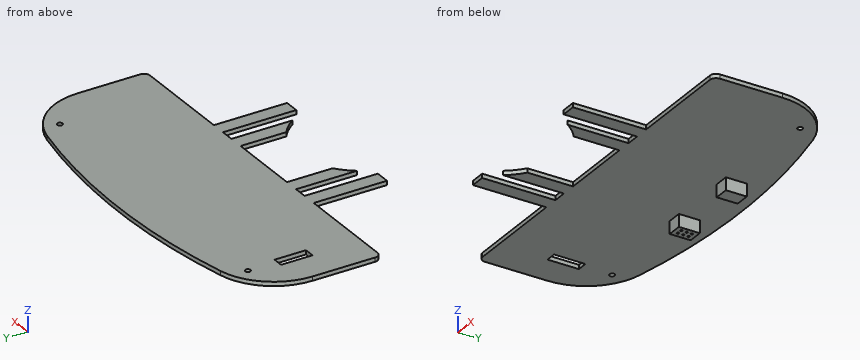
```python
from build123d import *

# Parameters (mm, degrees)
PAD019_DEPTH    = 2
FILLET016_R     = 30
SKETCH039_R     = 1.25
POCKET019_DEPTH = 2.001
FILLET017_R     = 3
SKETCH041_W     = 5
SKETCH041_H     = 15
POCKET020_DEPTH = 5
SKETCH042_W     = 7
SKETCH042_H     = 10
PAD020_DEPTH    = 6
SKETCH044_R     = 0.5
POCKET021_DEPTH = 6
SKETCH045_R     = 30
POCKET022_DEPTH = 7


with BuildPart() as part:
    # Sketch038 → Pad019 (new body)
    with BuildSketch(Plane.XY):
        with BuildLine():
            Line((-90, -38.494821), (-90, 17.505179))
            ThreePointArc((90, 17.505179), (0, 30.6), (-90, 17.505179))
            Line((90, 17.505179), (90, -38.494821))
            Line((90, -38.494821), (38.25, -38.494821))
            Line((38.25, -73.494821), (38.25, -38.494821))
            Line((31.25, -73.494821), (38.25, -73.494821))
            Line((31.25, -38.494821), (31.25, -73.494821))
            Line((24.75, -38.494821), (31.25, -38.494821))
            Line((24.75, -73.494821), (24.75, -38.494821))
            Line((17.75, -73.494821), (24.75, -73.494821))
            Line((17.75, -38.494821), (17.75, -73.494821))
            Line((-17.75, -38.494821), (17.75, -38.494821))
            Line((-17.75, -73.494821), (-17.75, -38.494821))
            Line((-24.75, -73.494821), (-17.75, -73.494821))
            Line((-24.75, -38.494821), (-24.75, -73.494821))
            Line((-31.25, -38.494821), (-24.75, -38.494821))
            Line((-31.25, -73.494821), (-31.25, -38.494821))
            Line((-38.25, -73.494821), (-31.25, -73.494821))
            Line((-38.25, -38.494821), (-38.25, -73.494821))
            Line((-38.25, -38.494821), (-90, -38.494821))
        make_face()
    extrude(amount=PAD019_DEPTH)

    # Fillet016
    fillet016_edges = [part.edges().sort_by_distance(p)[0] for p in [
        (90, 17.505179, 1),
        (-90, 17.505179, 1),
    ]]
    fillet(fillet016_edges, radius=FILLET016_R)

    # Sketch039 (on Face2 of Fillet016) → Pocket019 (cut, through all)
    with BuildSketch(Plane(origin=(0, 0, 0), x_dir=(1, 0, 0), z_dir=(0, 0, -1))):
        with Locations((-72, -14)):
            Circle(SKETCH039_R)
        with Locations((72, -14)):
            Circle(SKETCH039_R)
    extrude(amount=-POCKET019_DEPTH, mode=Mode.SUBTRACT)

    # Fillet017
    fillet017_edges = [part.edges().sort_by_distance(p)[0] for p in [
        (-90, -38.494821, 1),
        (90, -38.494821, 1),
    ]]
    fillet(fillet017_edges, radius=FILLET017_R)

    # Sketch041 (on Face2 of Fillet017) → Pocket020 (cut)
    with BuildSketch(Plane(origin=(0, 0, 0), x_dir=(1, 0, 0), z_dir=(0, 0, -1))):
        with Locations((-72.5, 7.5)):
            Rectangle(SKETCH041_W, SKETCH041_H)
    extrude(amount=-POCKET020_DEPTH, mode=Mode.SUBTRACT)

    # Sketch042 (on Face2 of Pocket020) → Pad020 (join)
    with BuildSketch(Plane(origin=(0, 0, 0), x_dir=(1, 0, 0), z_dir=(0, 0, -1))):
        with Locations((18, -15)):
            Rectangle(SKETCH042_W, SKETCH042_H)
        with Locations((-18, -15)):
            Rectangle(SKETCH042_W, SKETCH042_H)
    extrude(amount=PAD020_DEPTH)

    # Sketch044 (on Face42 of Pad020) → Pocket021 (cut)
    with BuildSketch(Plane(origin=(0, 0, -6), x_dir=(1, 0, 0), z_dir=(0, 0, -1))):
        with Locations((-19.2, -12.5)):
            Circle(SKETCH044_R)
        with Locations((-16.65, -12.5)):
            Circle(SKETCH044_R)
        with Locations((-19.2, -15.05)):
            Circle(SKETCH044_R)
        with Locations((-16.65, -15.05)):
            Circle(SKETCH044_R)
        with Locations((-19.2, -17.6)):
            Circle(SKETCH044_R)
        with Locations((-16.65, -17.6)):
            Circle(SKETCH044_R)
    extrude(amount=-POCKET021_DEPTH, mode=Mode.SUBTRACT)

    # Sketch045 (on Face2 of Pocket021) → Pocket022 (cut)
    with BuildSketch(Plane(origin=(0, 0, 0), x_dir=(1, 0, 0), z_dir=(0, 0, -1))):
        with Locations((0, 84.494821)):
            Circle(SKETCH045_R)
    extrude(amount=-POCKET022_DEPTH, mode=Mode.SUBTRACT)


with BuildPart() as part_1:
    # Body014 placement: moved
    add(part.part.moved(Location((0, 0, -2))))


solid = part_1.part
```
CAD build for the part. Positions are in the model's coordinates, mm. Round coordinates to 2 decimals unless told otherwise and drop trailing zeros. Order: outer loops, then holes, each group sorted by start corner. A loop starts at its lowest first (then second) coordinate and runs counter-clockwise, first axis right, second up.
Item 1: Saw through at C-C on x = 10. Write the cut outline in (y, z), then the cut area to 3 significant figures.
Item 2: Saw through at B-B on z = -4. Write the cut outline in (x, y).
Item 3: Pin check, flat tips, straight feed: pin 1 (1 mm diameter, centred on y = -51, z = -1.5, fed in from -X); pin 2 (0.8 mm diameter, centred on x = -16.5, y = 17.5, fed in from -Z); pin 3 (0.6 mm diameter, centred on x = 29.5, z = -1, fed in from -Y); pin 4 (3 mm diameter, centred on y = 3, z = -2.5, fed in from +X). Stop position of each tip, or through.
Item 4: Probe line 1 along X through (y, z) = (12.5, -6.15); line 2 along Y through (x, z) = (-16.65, -5.5); line 3 along X through (y, z) = (-41, -0.25). List the from-to ranges inside material, lowest first.
Item 5: Saw through at A-A on y = -9. Write the cut outline in (x, z).
Reported:
1. outline: (-38.49, -2) - (30.44, -2) - (30.44, 0) - (-38.49, 0) - close
1. area: 138 mm2
2. outline: (-21.5, 10) - (-14.5, 10) - (-14.5, 20) - (-21.5, 20) - close; (14.5, 10) - (21.5, 10) - (21.5, 20) - (14.5, 20) - close; hole circle Ø1 at (-19.2, 12.5); hole circle Ø1 at (-19.2, 15.05); hole circle Ø1 at (-19.2, 17.6); hole circle Ø1 at (-16.65, 12.5); hole circle Ø1 at (-16.65, 15.05); hole circle Ø1 at (-16.65, 17.6)
3. pin 1: stops at x = -38.25
3. pin 2: stops at z = -8
3. pin 3: stops at y = -38.49
3. pin 4: stops at x = 89.08
4. line 1: x = -21.5 to -19.7, -18.7 to -17.15, -16.15 to -14.5, 14.5 to 21.5
4. line 2: y = 10 to 12, 13 to 14.55, 15.55 to 17.1, 18.1 to 20
4. line 3: x = -38.25 to -31.25, -24.75 to -17.75, 17.75 to 24.75, 31.25 to 38.25
5. outline: (-90, -2) - (-75, -2) - (-75, 0) - (-90, 0) - close; (-70, -2) - (90, -2) - (90, 0) - (-70, 0) - close
